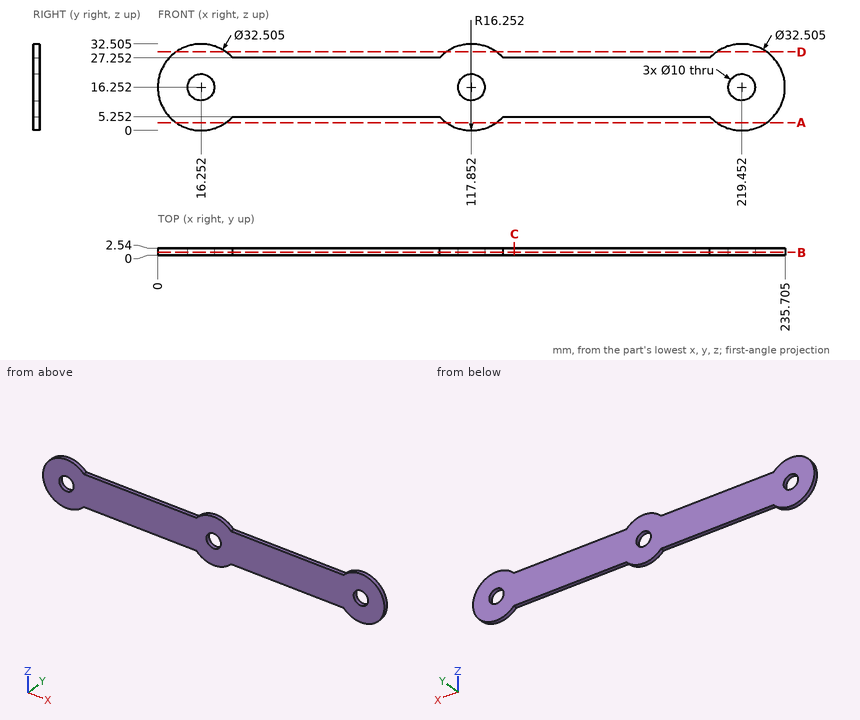
Part print with two shaded views. Sizes in mm from the minimum x, y, z corner. Coordinates: 2 decimals unless noted, no trailing zeros. Order: outer loops, then holes, each group sorted by start corner. A loop starts at its lowest first (then second) coordinate and runs counter-clockwise, first axis right, second up. Notation, with made-up numbers: (39.5, -38.75) - (62.5, -38.75) arc R32 ccw to (62.5, -6.75) - close; hole circle Ø8 at (-23, 26.25). An arc over 180 degrees is marked (long way). Answer in a Markdown table with one row per item.
1. Flat gauge pins, fed straight in: P1, Ø6, axis at x = 117.85, z = 16.25, coming from the +Y side; P2, Ø1.3, axis at x = 59.5, y = 1.5, coming from the +Z side; P3, Ø1, axis at x = 55.5, y = 1, coming from the -Z side; P4, Ø1.5, axis at y = 2, z = 12, coming from the +X side. Where does each tip first touch, or does it go through?
Answer:
| item | result |
|---|---|
| P1 | through |
| P2 | z = 27.25 |
| P3 | z = 5.25 |
| P4 | x = 235.32 |
2. Slice it at C-C, the plane x = 134. List the corners of the cut face in (y, z).
Answer:
| item | result |
|---|---|
| outline | (0, 5.25) - (2.54, 5.25) - (2.54, 27.25) - (0, 27.25) - close |
3. Slice it at D-D, the plane z = 29.5. List the corners of the cut face in (x, y).
Answer:
| item | result |
|---|---|
| outline | (6.84, 0) - (25.67, 0) - (25.67, 2.54) - (6.84, 2.54) - close; (108.44, 0) - (127.27, 0) - (127.27, 2.54) - (108.44, 2.54) - close; (210.04, 0) - (228.87, 0) - (228.87, 2.54) - (210.04, 2.54) - close |
4. Drill centre lines: L1, parallel to X at y = 2.45, z = 19 (1 decimal); L2, parallel to X at y = 1.5, z = 29 (1 decimal); L3, parallel to X at y = 1.35, z = 14 (1 decimal). Where is each one in solid material? Low to high. Write a range as from..to.
Answer:
| item | result |
|---|---|
| L1 | 0.2..12.1, 20.4..113.7, 122..215.3, 223.6..235.5 |
| L2 | 6.2..26.3, 107.8..127.9, 209.4..229.5 |
| L3 | 0.2..11.8, 20.7..113.4, 122.3..215, 223.9..235.5 |
5. Slice it at B-B, the plane y = 1.1. List the corners of the cut face in (x, z) (1 decimal).
Answer:
| item | result |
|---|---|
| outline | (28.2, 5.3) - (105.9, 5.3) arc R16.3 ccw to (129.8, 5.3) - (207.5, 5.3) arc R16.3 ccw (long way) to (207.5, 27.3) - (129.8, 27.3) arc R16.3 ccw to (105.9, 27.3) - (28.2, 27.3) arc R16.3 ccw (long way) to start; hole circle Ø10 at (16.3, 16.3); hole circle Ø10 at (117.9, 16.3); hole circle Ø10 at (219.5, 16.3) |
6. Slice it at A-A, the plane z = 3. List the corners of the cut face in (x, y).
Answer:
| item | result |
|---|---|
| outline | (6.84, 0) - (25.66, 0) - (25.66, 2.54) - (6.84, 2.54) - close; (108.44, 0) - (127.26, 0) - (127.26, 2.54) - (108.44, 2.54) - close; (210.04, 0) - (228.86, 0) - (228.86, 2.54) - (210.04, 2.54) - close |
